Geometry: final body of the model. Coordinates: model frame, mm. Face numbers are marked on the shaded views. A direction names the side the tool comes from. Give positions to 0.01 mm unless a question says otherwise; leave off trailing zeros. Write each loop counter-clockwise with the first axis right and the second up, starting at its lowest first coordinate (ties: lowest second). Pieces come first, ordered by that corner, then holes. Notation, with made-up numbers: (22, 53) -> (64, 53) arc R25 cw to (64, 70) -> close; hole circle Ø11 at (44, -19). An arc over 180 degrees is marked (long way). Use CSV: the item, a comma, the result in double quotes. Start each with the question number.
1) Contact query for flat-ended pins moving along their axis: P1, Ø5, axis at x = -6.5, y = -6.5, coming from the +Z side; P2, Ø1.8, axis at x = 13.42, y = -7.75, coming from the +Z side; P3, Ø12, axis at y = 9, z = -6, coming from the -X side. Output: stop coordinate, or through.
2) Set-up query: the marked faces 1, 2 and 3. Return all of +Z, -Z, +X, -X, +Y, -Y with unobstructed straight access to the full face (end or side cutting, diameter ignored); none if empty.
3) Section B-B (x = 0). Output: boundary loops of the cut face in (y, z), plus the area to 3 significant figures.
4) Section A-A (y = 1.5). Output: boundary loops of the cut face in (x, z).
5) Section C-C (z = 9.5). Output: boundary loops of the cut face in (x, y).
6) Section D-D (y = -12.5). Output: boundary loops of the cut face in (x, z).
7) Material intervals for line 1 (Y direction, x = 0, z = 23.15); line 2 (Z direction, x = 2, y = -7.5); line 3 (Z direction, x = 12, y = 8), sorted ascending. Write a range as [from, to].
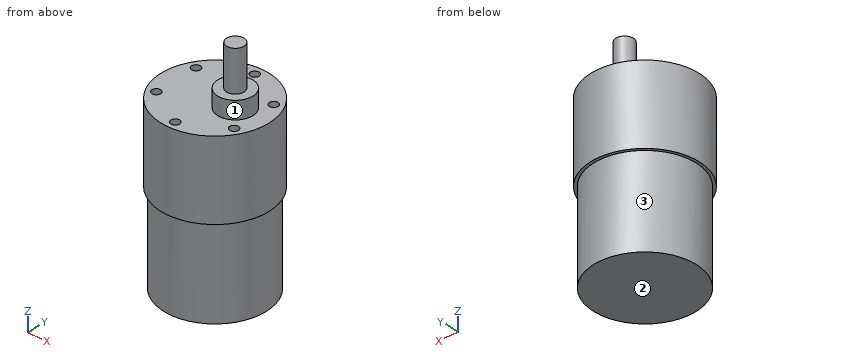
```python
from build123d import *

# Parameters (mm, degrees)
F0_R     = 18.5
F0_R_2   = 17.5
F1_DEPTH = 27
F2_DEPTH = 31
F3_R     = 1.5
F4_DEPTH = 5
F3_R_2   = 6
F3_R_3   = 3
F5_DEPTH = 6
F6_DEPTH = 20


with BuildPart() as f1:
    # F0 (on Top) → F1 (new body)
    with BuildSketch(Plane.XY):
        Circle(F0_R)
        Circle(F0_R_2, mode=Mode.SUBTRACT)
        Circle(F0_R_2)
    extrude(amount=F1_DEPTH)

    # F0 (on Top) → F2 (join)
    with BuildSketch(Plane.XY):
        Circle(F0_R_2)
    extrude(amount=-F2_DEPTH)

    # F3 (on face) → F4 (cut)
    with BuildSketch(Plane.XY.offset(27)):
        with Locations((0, 15.5)):
            Circle(F3_R)
        with Locations((13.4233937587, 7.75)):
            Circle(F3_R)
        with Locations((13.4233937587, -7.75)):
            Circle(F3_R)
        with Locations((0, -15.5)):
            Circle(F3_R)
        with Locations((-13.4233937587, -7.75)):
            Circle(F3_R)
        with Locations((-13.4233937587, 7.75)):
            Circle(F3_R)
    extrude(amount=-F4_DEPTH, mode=Mode.SUBTRACT)

    # F3 (on face) → F5 (join)
    with BuildSketch(Plane.XY.offset(27)):
        with Locations((7, 0)):
            Circle(F3_R_2)
        with Locations((7, 0)):
            Circle(F3_R_3, mode=Mode.SUBTRACT)
    extrude(amount=F5_DEPTH)

    # F6 (add): a face of the model
    f6_faces = [f1.faces().sort_by_distance(p)[0] for p in [
        (7, 0, 27),
    ]]
    extrude(f6_faces, amount=F6_DEPTH)


solid = f1.part
```
Answers follow:
1,P1,"stops at z = 27"
1,P2,"stops at z = 22"
1,P3,"stops at x = -17.24"
2,face 1,"+Z"
2,face 2,"-Z, +X, -X, +Y, -Y"
2,face 3,"-Z"
3,outline,"(-18.5, 0) -> (-17.5, 0) -> (-17.5, -31) -> (17.5, -31) -> (17.5, 0) -> (18.5, 0) -> (18.5, 27) -> (17, 27) -> (17, 22) -> (14, 22) -> (14, 27) -> (-14, 27) -> (-14, 22) -> (-17, 22) -> (-17, 27) -> (-18.5, 27) -> close"
3,area,"2,050 mm^2"
4,outline,"(-18.44, 0) -> (-17.44, 0) -> (-17.44, -31) -> (17.44, -31) -> (17.44, 0) -> (18.44, 0) -> (18.44, 27) -> (12.81, 27) -> (12.81, 33) -> (9.6, 33) -> (9.6, 47) -> (4.4, 47) -> (4.4, 33) -> (1.19, 33) -> (1.19, 27) -> (-18.44, 27) -> close"
5,outline,"circle Ø37 at (0, 0)"
6,outline,"(-13.64, 0) -> (-12.25, 0) -> (-12.25, -31) -> (12.25, -31) -> (12.25, 0) -> (13.64, 0) -> (13.64, 27) -> (-13.64, 27) -> close"
7,line 1,"y = [-18.5, -17], [-14, 14], [17, 18.5]"
7,line 2,"z = [-31, 27]"
7,line 3,"z = [-31, 22]"
